Print and shaded views of the part. All mm, measured from the part's lowest x, y and z. A direction names the side the tool comes from. Round coordinates to 2 decimals unless told otherwise and drop trailing zeros. Write each loop counter-clockwise with the first axis right and the second up, starting at its lowest first coordinate (ties: lowest second). Pieces come first, ordered by that corner, then holes. Notation, with made-up numbers: (12, -30) -> (28, -30) arc R37 ccw to (28, 6) -> close; hole circle Ø5 at (33, 42.5). An arc over 180 degrees is marked (long way). Use CSV: the item, a comma, the result in double quotes. Start each with the question number.
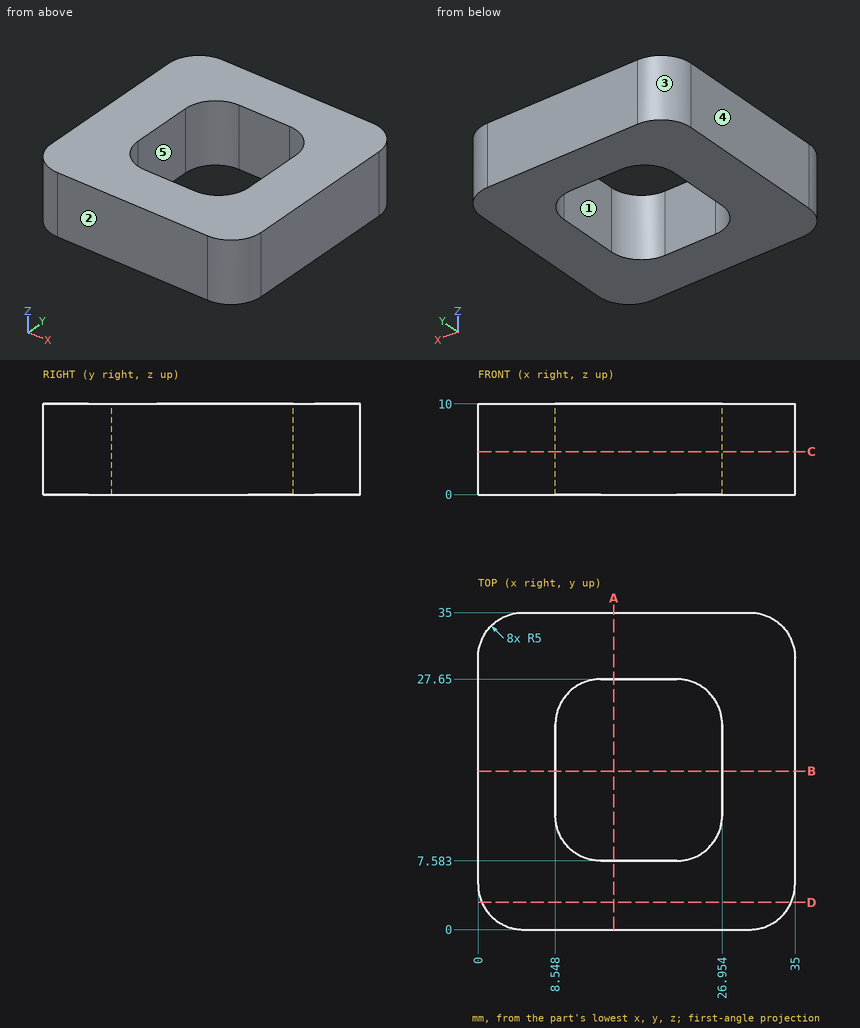
1. Band-saw the part on A-A (x = 15). List the corners of the cut face in (y, z).
2. Which spindle directions (+Z, -Z, +X, -X, +Y, -Y) get a long thin tool onto all of the face, cutting with end or side? Do the marked faces 1 and 2. Say none if no direction does.
3. Band-saw the part on D-D (y = 3). List the corners of the cut face in (x, z), then the cut area to 3 significant figures.
4. Drill centre lines: line 1 along X through (y, z) = (20.5, 3); line 2 along Y through (x, z) = (14, 1.5); line 3 along X through (y, z) = (26, 3.5) (1 decimal). Where is each one in solid material? Low to high. Write a range as [from, to].
5. Flat gauge pin, fed straight in: pin 1 (1.5 mm diameter, centred on y = 3.5, z = 7.5, fed in from -X). Where does the tip first touch, or does it go through?
6. Band-saw the part on B-B (y = 17.5). List the corners of the cut face in (x, z).
7. Pull direction Y, two halves, no side cores. Call the marked faces 3, 4 and 5: released by +Y, released by -Y, zero draft, split by the parting line, or undercut.
8. Band-saw the part on C-C (z = 4.75). List the corners of the cut face in (x, y).
Answers below:
1,outline,"(0, 0) -> (7.58, 0) -> (7.58, 10) -> (0, 10) -> close; (27.65, 0) -> (35, 0) -> (35, 10) -> (27.65, 10) -> close"
2,face 1,"+Z, -Z"
2,face 2,"+Z, -Z, +X, -X, -Y"
3,outline,"(0.42, 0) -> (34.58, 0) -> (34.58, 10) -> (0.42, 10) -> close"
3,area,"342 mm^2"
4,line 1,"x = [0, 8.55], [26.95, 35]"
4,line 2,"y = [0, 7.58], [27.65, 35]"
4,line 3,"x = [0, 9.8], [25.7, 35]"
5,pin 1,"stops at x = 0.06"
6,outline,"(0, 0) -> (8.55, 0) -> (8.55, 10) -> (0, 10) -> close; (26.95, 0) -> (35, 0) -> (35, 10) -> (26.95, 10) -> close"
7,face 3,"released by +Y"
7,face 4,"zero draft"
7,face 5,"undercut"
8,outline,"(0, 5) arc R5 ccw to (5, 0) -> (30, 0) arc R5 ccw to (35, 5) -> (35, 30) arc R5 ccw to (30, 35) -> (5, 35) arc R5 ccw to (0, 30) -> close; hole (8.55, 12.58) arc R5 ccw to (13.55, 7.58) -> (21.95, 7.58) arc R5 ccw to (26.95, 12.58) -> (26.95, 22.65) arc R5 ccw to (21.95, 27.65) -> (13.55, 27.65) arc R5 ccw to (8.55, 22.65) -> close"
